```python
from build123d import *

# Parameters (mm, degrees)
SKETCH1_R                = 11.5062
BOSS_EXTRUDE1_DEPTH      = 4.7625
BOSS_EXTRUDE1_DEPTH_BACK = 4.7625
CUT_EXTRUDE1_START       = -4.7625
CUT_EXTRUDE1_DEPTH       = 1.5875
CUT_EXTRUDE2_START       = 3.175
CUT_EXTRUDE2_DEPTH       = 1.5875
FILLET1_R                = 1.5875


with BuildPart() as part:
    # Sketch1 → Boss-Extrude1 (new body, two sides)
    with BuildSketch(Plane.XY) as boss_extrude1_sk:
        with BuildLine():
            ThreePointArc((14.639156809, 1.110279863), (-4.45502565, 13.988937769), (-12.585193267, -7.559797873))
            ThreePointArc((-12.585193267, -7.559797873), (4.45502565, -13.988937769), (14.639156809, 1.110279863))
        make_face()
        Circle(SKETCH1_R, mode=Mode.SUBTRACT)
        with BuildLine():
            ThreePointArc((-12.585193267, -7.559797873), (4.45502565, -13.988937769), (14.639156809, 1.110279863))
            ThreePointArc((14.639156809, 1.110279863), (15.535368252, -3.075379389), (17.517315641, -6.869430374))
            Line((17.517315641, -6.869430374), (37.052935248, -34.429965394))
            Line((37.052935248, -34.429965394), (20.216142238, -46.364319477))
            Line((20.216142238, -46.364319477), (10.31875, -32.401239172))
            Line((10.31875, -32.401239172), (10.31875, -49.389319794))
            Line((10.31875, -49.389319794), (-10.31875, -49.389319794))
            Line((-10.31875, -49.389319794), (-10.31875, -15.734319794))
            ThreePointArc((-10.31875, -15.734319794), (-10.89585042, -11.492870345), (-12.585193267, -7.559797873))
        make_face()
        with BuildLine():
            ThreePointArc((20.774153775, -19.699685133), (13.028075711, -18.379797729), (11.708188308, -26.125875793))
            Line((11.708188308, -26.125875793), (18.134378968, -35.19184126))
            ThreePointArc((18.134378968, -35.19184126), (25.880457031, -36.511728663), (27.200344435, -28.7656506))
            Line((27.200344435, -28.7656506), (20.774153775, -19.699685133))
        make_face(mode=Mode.SUBTRACT)
        with BuildLine():
            ThreePointArc((5.55625, -27.958069794), (0, -22.401819794), (-5.55625, -27.958069794))
            Line((-5.55625, -27.958069794), (-5.55625, -39.070569794))
            ThreePointArc((-5.55625, -39.070569794), (0, -44.626819794), (5.55625, -39.070569794))
            Line((5.55625, -39.070569794), (5.55625, -27.958069794))
        make_face(mode=Mode.SUBTRACT)
    extrude(amount=BOSS_EXTRUDE1_DEPTH)
    extrude(boss_extrude1_sk.sketch, amount=-BOSS_EXTRUDE1_DEPTH_BACK)

    # Sketch2 → Cut-Extrude1 (cut)
    with BuildSketch(Plane.XY.offset(CUT_EXTRUDE1_START)):
        with BuildLine():
            Line((-10.31875, -15.734319794), (-10.31875, -49.389319794))
            Line((-10.31875, -49.389319794), (10.31875, -49.389319794))
            Line((10.31875, -49.389319794), (10.31875, -32.401239172))
            Line((10.31875, -32.401239172), (20.216142238, -46.364319477))
            Line((20.216142238, -46.364319477), (37.052935248, -34.429965394))
            Line((37.052935248, -34.429965394), (17.517315641, -6.869430374))
            ThreePointArc((17.517315641, -6.869430374), (15.535368252, -3.075379389), (14.639156809, 1.110279863))
            ThreePointArc((14.639156809, 1.110279863), (4.45502565, -13.988937769), (-12.585193267, -7.559797873))
            ThreePointArc((-12.585193267, -7.559797873), (-10.89585042, -11.492870345), (-10.31875, -15.734319794))
        make_face()
        with BuildLine():
            Line((-5.55625, -39.070569794), (-5.55625, -27.958069794))
            ThreePointArc((-5.55625, -27.958069794), (0, -22.401819794), (5.55625, -27.958069794))
            Line((5.55625, -27.958069794), (5.55625, -39.070569794))
            ThreePointArc((5.55625, -39.070569794), (0, -44.626819794), (-5.55625, -39.070569794))
        make_face(mode=Mode.SUBTRACT)
        with BuildLine():
            Line((18.134378968, -35.19184126), (11.708188308, -26.125875793))
            ThreePointArc((11.708188308, -26.125875793), (13.028075711, -18.379797729), (20.774153775, -19.699685133))
            Line((20.774153775, -19.699685133), (27.200344435, -28.7656506))
            ThreePointArc((27.200344435, -28.7656506), (25.880457031, -36.511728663), (18.134378968, -35.19184126))
        make_face(mode=Mode.SUBTRACT)
    extrude(amount=CUT_EXTRUDE1_DEPTH, mode=Mode.SUBTRACT)

    # Sketch2_6 → Cut-Extrude2 (cut)
    with BuildSketch(Plane.XY.offset(CUT_EXTRUDE2_START)):
        with BuildLine():
            Line((-10.31875, -15.734319794), (-10.31875, -49.389319794))
            Line((-10.31875, -49.389319794), (10.31875, -49.389319794))
            Line((10.31875, -49.389319794), (10.31875, -32.401239172))
            Line((10.31875, -32.401239172), (20.216142238, -46.364319477))
            Line((20.216142238, -46.364319477), (37.052935248, -34.429965394))
            Line((37.052935248, -34.429965394), (17.517315641, -6.869430374))
            ThreePointArc((17.517315641, -6.869430374), (15.535368252, -3.075379389), (14.639156809, 1.110279863))
            ThreePointArc((14.639156809, 1.110279863), (4.45502565, -13.988937769), (-12.585193267, -7.559797873))
            ThreePointArc((-12.585193267, -7.559797873), (-10.89585042, -11.492870345), (-10.31875, -15.734319794))
        make_face()
        with BuildLine():
            Line((-5.55625, -39.070569794), (-5.55625, -27.958069794))
            ThreePointArc((-5.55625, -27.958069794), (0, -22.401819794), (5.55625, -27.958069794))
            Line((5.55625, -27.958069794), (5.55625, -39.070569794))
            ThreePointArc((5.55625, -39.070569794), (0, -44.626819794), (-5.55625, -39.070569794))
        make_face(mode=Mode.SUBTRACT)
        with BuildLine():
            Line((18.134378968, -35.19184126), (11.708188308, -26.125875793))
            ThreePointArc((11.708188308, -26.125875793), (13.028075711, -18.379797729), (20.774153775, -19.699685133))
            Line((20.774153775, -19.699685133), (27.200344435, -28.7656506))
            ThreePointArc((27.200344435, -28.7656506), (25.880457031, -36.511728663), (18.134378968, -35.19184126))
        make_face(mode=Mode.SUBTRACT)
    extrude(amount=CUT_EXTRUDE2_DEPTH, mode=Mode.SUBTRACT)

    # Fillet1
    fillet1_edges = [part.edges().sort_by_distance(p)[0] for p in [
        (-10.31875, -49.389319794, 0),
        (10.31875, -49.389319794, 0),
        (10.31875, -32.401239172, 0),
        (20.216142238, -46.364319477, 0),
        (37.052935248, -34.429965394, 0),
    ]]
    fillet(fillet1_edges, radius=FILLET1_R)


solid = part.part
```
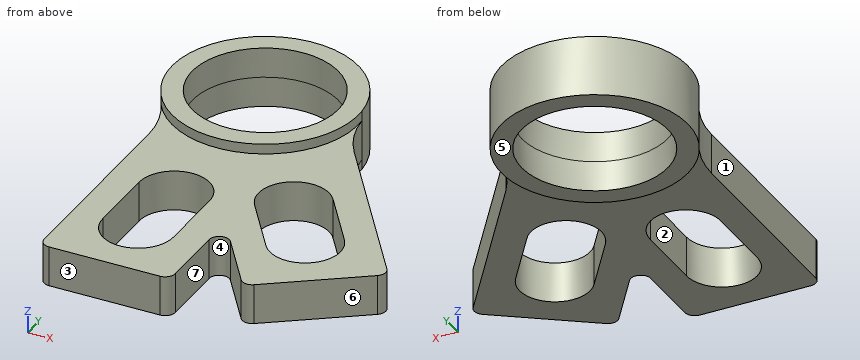
Part model, mm, in its own coordinate system. Face numbers are marked on the shaded views. A direction names the side the tool comes from. Round coordinates to 2 decimals unless told otherwise and drop trailing zeros. Order: outer loops, then holes, each group sorted by start corner. A loop starts at its lowest first (then second) coordinate and runs counter-clockwise, first axis right, second up. Notation, with made-up numbers: M 32.25,52.5 L 77.25,52.5 A25 ccw 77.25,91.5 Z; hole C -17.5,22.5 d2. An arc over 180 degrees is marked long. Answer in a Markdown table with one row per item. Add a question column.
Q1. Cut at B-B on x = 0. Give the cut face in (y, z) (1 decimal), and give its area (3 significant figures).
Q2. 3-axis set-ups, long thin cutter, end or side, ignore diameter. For the marked faces 1, 2 and 3: which of +Z, -Z, +X, -X, +Y, -Y reach the whole face in a straight line?
Q3. Cut at A-A on y = -30.5. Give the cut face in (x, z) (3 decimals), and give its area (3 significant figures).
Q4. Pin check, flat tips, straight feed: pin 1 (1 mm diameter, centred on y = -21, z = -2.5, fed in from +X); pin 2 (3 mm diameter, centred on x = -4.5, z = 3, fed in from +Y); pin 3 (6 mm diameter, centred on x = 19, y = -23, fed in from +Z); pin 4 (1 mm diameter, centred on y = -41.5, z = -2, fed in from +X). Stop position of each tip, or through.
Q5. Wall check: L1, parallel to Y at x = 0, z = 1.3; L2, parallel to X at y = -40, z = -1; L3, parallel to X at y = -2, z = -1.5. Give the ranges that are in metal, low to high. Write a range as from..to.
Q6. Mould opens along X. For the marked faces 4, 5, 6 and 7 say: +X half, -X half, draft (parallel to the pull), parting line (faces both ways), or undercut.
Q7. Cut at C-C on z = -2.25. Give the number of separate pieces and of enclosed holes in the cut face, and give its area (3 significant figures).
Established:
| question | item | result |
|---|---|---|
| 1 | outline | M -49.4,-3.2 L -44.6,-3.2 L -44.6,3.2 L -49.4,3.2 Z; M -22.4,-3.2 L -14.7,-3.2 L -14.7,-4.8 L -11.5,-4.8 L -11.5,4.8 L -14.7,4.8 L -14.7,3.2 L -22.4,3.2 Z; M 11.5,-4.8 L 14.7,-4.8 L 14.7,4.8 L 11.5,4.8 Z |
| 1 | area | 140 mm2 |
| 2 | face 1 | +Z, -Z, -X, -Y |
| 2 | face 2 | +Z, -Z |
| 2 | face 3 | +Z, -Z, +X, -X, -Y |
| 3 | outline | M -10.319,-3.175 L -5.556,-3.175 L -5.556,3.175 L -10.319,3.175 Z; M 5.556,-3.175 L 14.809,-3.175 L 14.809,3.175 L 5.556,3.175 Z; M 28.023,-3.175 L 34.267,-3.175 L 34.267,3.175 L 28.023,3.175 Z |
| 3 | area | 129 mm2 |
| 4 | pin 1 | stops at x = 27.89 |
| 4 | pin 2 | stops at y = 14.37 |
| 4 | pin 3 | passes through |
| 4 | pin 4 | stops at x = 27.78 |
| 5 | L1 | y = -49.39..-44.63, -22.4..-11.51, 11.51..14.68 |
| 5 | L2 | x = -10.32..-5.48, 5.48..10.32, 15.7..29.19 |
| 5 | L3 | x = -14.54..-11.33, 11.33..15.19 |
| 6 | face 4 | undercut |
| 6 | face 5 | draft |
| 6 | face 6 | +X half |
| 6 | face 7 | undercut |
| 7 | separate pieces | 1 |
| 7 | enclosed holes | 3 |
| 7 | area | 1,190 mm2 |
